Design review of the part built by this model. Coordinates are the model's own, in mm. A direction names the side the tool comes from. Coordinates: 2 decimals unless noted, no trailing zeros. Loops run counter-clockwise (first coordinate to the right, second up) from the corner with the lowest first, then second, coordinate; pieces in that order, holes last.
Q1. Machinability: for faces 5 (the face through (0.15, -3.44, -5.22)), 6 (the face through (0, -0.381, -5)), which of the approach directions +Z, -Z, +X, -X, +Y, -Y give a long, thin tool a straight path to every point of the face, cutting with its end or side? Answer none if there is none.
Q2. Add section D-D on z = -3.75. Give the boundary of the cut face in (x, y) (3 decimals), and give its area (3 significant figures).
Q3. Add section B-B on z = -0.25. Give the boundary of the cut face in (x, y) (3 decimals), and give its area (3 significant figures).
Q4. Draft analysis for pull direction X (two halves, no side actions). For faces 1 (the face through (-1.905, 0, 4)), 2 (the face through (0, 0.381, -5)), 3 (the face through (0.15, 3.35, -5.22)), 4 (the face through (1.905, 0, 4)), state which applies: released by +X, released by -X, zero draft, split by the parting line, or undercut.
Q5. Add section A-A on y = 1. Give the boundary of the cut face in (x, z) (3 decimals).
Q6. For P1, Ø1.9, axis at x = 0, z = -5.5, coming from the +Y side; P2, Ø1.2, axis at x = 0, z = -5.71, coming from the -Y side; P3, Ø1, axis at x = 0, z = -5.5, coming from the -Y side, all flat-tipped, find the tip position at first contact; note any pin that passes through.
Q7. Wall thickness on probe 1 along Z at (x, y) = (0, 2.25); probe 2 along Z at (x, y) = (0, 2.75); probe 3 along Z at (x, y) = (1.45, 1): over which ranges is each line inside the solid? List them lowest first.
Q8. Add section C-C on x = 0. Give the boundary of the cut face in (y, z) (3 decimals).
```python
from build123d import *

# Parameters (mm, degrees)
SKETCH1_R               = 8.255
SKETCH1_R_2             = 3.175
BOSS_EXTRUDE1_DEPTH     = 1.905
SKETCH3_W               = 3.81
SKETCH3_H               = 8.255
CUT_EXTRUDE1_DEPTH      = 0.381
CUT_EXTRUDE2_DEPTH      = 12.828739366
CUT_EXTRUDE2_DEPTH_BACK = 12.828739366
SKETCH4_R               = 0.508


with BuildPart() as part:
    # Sketch1 → Boss-Extrude1 (new, symmetric)
    with BuildSketch(Plane(origin=(0, 0, 0), x_dir=(0, 0, -1), z_dir=(1, 0, 0))):
        with Locations(Location((0, 0, 0), (0, 0, 180))):
            Circle(SKETCH1_R)
        with Locations(Location((0, 0, 0), (0, 0, 180))):
            Circle(SKETCH1_R_2, mode=Mode.SUBTRACT)
    extrude(amount=BOSS_EXTRUDE1_DEPTH, both=True)

    # Sketch3 → Cut-Extrude1 (cut, symmetric)
    with BuildSketch(Plane(origin=(0, 0, 0), x_dir=(1, 0, 0), z_dir=(0, 1, 0))):
        with Locations((0, 4.1275)):
            Rectangle(SKETCH3_W, SKETCH3_H)
    extrude(amount=CUT_EXTRUDE1_DEPTH, both=True, mode=Mode.SUBTRACT)

    # Sketch4 → Cut-Extrude2 (cut, two sides: drawn at the far end of the back side and taken through both)
    with BuildSketch(Plane(origin=(0, 0, 0), x_dir=(1, 0, 0), z_dir=(0, 1, 0)).offset(-CUT_EXTRUDE2_DEPTH_BACK)):
        with Locations(Location((0, 5.706203005, 0), (0, 0, 270))):
            Circle(SKETCH4_R)
    extrude(amount=CUT_EXTRUDE2_DEPTH + CUT_EXTRUDE2_DEPTH_BACK, mode=Mode.SUBTRACT)


solid = part.part
```
Entries:
1. face 5: +Y, -Y
1. face 6: -Z, +X, -X
2. outline: (-1.905, -7.354) - (1.905, -7.354) - (1.905, -0.381) - (-1.905, -0.381) - close; (-1.905, 0.381) - (1.905, 0.381) - (1.905, 7.354) - (-1.905, 7.354) - close
2. area: 53.1 mm2
3. outline: (-1.905, -8.251) - (1.905, -8.251) - (1.905, -3.165) - (-1.905, -3.165) - close; (-1.905, 3.165) - (1.905, 3.165) - (1.905, 8.251) - (-1.905, 8.251) - close
3. area: 38.8 mm2
4. face 1: released by -X
4. face 2: zero draft
4. face 3: undercut
4. face 4: released by +X
5. outline: (-1.905, -8.194) - (1.905, -8.194) - (1.905, -3.013) - (-1.905, -3.013) - close; (-1.905, 3.013) - (1.905, 3.013) - (1.905, 8.194) - (-1.905, 8.194) - close; hole circle Ø1.016 at (0, -5.706)
6. P1: stops at y = 6.89
6. P2: stops at y = -6.48
6. P3: stops at y = -6.57
7. probe 1: z = -7.94 to -6.21, -5.2 to -2.24, 2.24 to 7.94
7. probe 2: z = -7.78 to -6.21, -5.2 to -1.59, 1.59 to 7.78
7. probe 3: z = -8.19 to -3.01, 3.01 to 8.19
8. outline: (-6.413, -5.198) - (-0.381, -5.198) - (-0.381, -3.152) arc R3.175 cw (long way) to (0.381, -3.152) - (0.381, -5.198) - (6.413, -5.198) arc R8.255 ccw (long way) to start; (-5.434, -6.214) arc R8.255 ccw to (-0.381, -8.246) - (-0.381, -6.214) - close; (0.381, -8.246) arc R8.255 ccw to (5.434, -6.214) - (0.381, -6.214) - close
